For this review, take the finished solid that the model builds, in its own axes (mm). A direction names the side the tool comes from. Give positions to 0.01 mm unless a question says otherwise; leave off trailing zeros. Write each loop counter-clockwise with the first axis right and the second up, starting at its lowest first coordinate (ties: lowest second). Pieces come first, ordered by that corner, then holes. Notation, with made-up numbers: M -33,-12.75 L 24,-12.75 A5 cw 24,-6.75 Z; hole C 37,87 d2. An arc over 180 degrees is marked long. One line per item, written item: value. Start each with the question number.
Item 1: Mouldability with a two-part tool opening along X and no side actions: class faces 1 (the face through (-256.7, 5.1, 83.7)), 2 (the face through (231.62, 16.99, 93.29)), 3 (the face through (23, 0, 4)) as released by +X, released by -X, zero draft, split by the parting line, or undercut.
Item 2: Clearance check with flat-ended pins moving along their axes: pin 1 Ø16.5 at (x, z) = (-234.5, 78.5) entering from +Y; pin 2 Ø5 at (x, y) = (-204.5, 69) entering from -Z; pin 3 Ø14.5 at (x, z) = (-164, 57) entering from +Y; pin 4 Ø11.5 at (x, z) = (-143.49, -197.5) entering from -Y. State where each tip first meets the part, or that it passes through.
Item 3: Tool access review of faces 4 (the face through (139, 20, -191)), 5 (the face through (111.363, 125.695, -124.104)), 6 (the face through (152.443, 125.695, 67.563)): name each direction out of +Z, -Z, +X, -X, +Y, -Y from which nothing blocks a thin tool from reaching the whole face with its end or side.
Item 4: To check wall thickness, follow probe 1 along X at (y, z) = (11.5, 0); probe 2 along Z at (x, y) = (114.5, 27); probe 3 along X at (y, z) = (50, 0). State the ranges of each line that lie inside material, in increasing order.
Item 5: Consider section A-A, the plane z = 0. Write out the cut boundary in (x, y).
Item 6: Consider section B-B, the plane x = 47. Write out the cut boundary in (y, z), and give its area (3 significant figures).
```python
from build123d import *

# Parameters (mm, degrees)
CROQUIS4_R              = 150
SALIENTE_EXTRUIR3_DEPTH = 150
CROQUIS7_R              = 130
CORTAR_EXTRUIR1_DEPTH   = 130
SALIENTE_EXTRUIR5_DEPTH = 20
REDONDEO1_R             = 10
MATRIZC1_COUNT          = 5
REDONDEO1_OF_MATRIZC1_R = 10
CROQUIS13_R             = 20
CORTAR_EXTRUIR2_DEPTH   = 406.648747611


with BuildPart() as part:
    # Croquis4 → Saliente-Extruir3 (new body)
    with BuildSketch(Plane(origin=(0, 0, 0), x_dir=(1, 0, 0), z_dir=(0, 1, 0))):
        with Locations(Location((0, 0, 0), (0, 0, 270))):
            Circle(CROQUIS4_R)
    extrude(amount=SALIENTE_EXTRUIR3_DEPTH)

    # Croquis7 → Cortar-Extruir1 (cut)
    with BuildSketch(Plane(origin=(0, 150, 0), x_dir=(1, 0, 0), z_dir=(0, 1, 0))):
        with Locations(Location((0, 0, 0), (0, 0, 270))):
            Circle(CROQUIS7_R)
    extrude(amount=-CORTAR_EXTRUIR1_DEPTH, mode=Mode.SUBTRACT)

    # Croquis8 → Saliente-Extruir5 (add, symmetric)
    with BuildSketch(Plane(origin=(0, 0, 0), x_dir=(0, 0, -1), z_dir=(1, 0, 0))):
        Polygon((-190.212550173, 128.702405531), (-220, 20), (-270, 20), (-270, 0), (-141.546888578, 0), (-141.546888578, 128.702405531), align=None)
    saliente_extruir5 = extrude(amount=SALIENTE_EXTRUIR5_DEPTH, both=True)

    # Redondeo1
    redondeo1_edges = [part.edges().sort_by_distance(p)[0] for p in [
        (20, 128.702405531, 169.436618823),
        (20, 74.351202766, 205.106275086),
        (20, 20, 245),
        (-20, 128.702405531, 169.436618823),
        (0, 128.702405531, 190.212550173),
        (0, 20, 270),
        (-20, 20, 245),
        (0, 20, 220),
        (-20, 74.351202766, 205.106275086),
    ]]
    fillet(redondeo1_edges, radius=REDONDEO1_R)

    # Croquis12 → Refrentado para tornillo con cabeza plana de M81 (revolve, cut)
    with BuildSketch(Plane(origin=(0, 20, 244.12063984), x_dir=(0, 0, 1), z_dir=(1, 0, 0))):
        Polygon((0, 0), (0, 20), (5, 20), (5, 5), (7.5, 5), (7.5, 0.025), (7.525, 0), align=None)
    refrentado_para_tornillo_con_cabeza_plan = revolve(axis=Axis((0, 26.35, 244.12063984), (0, -1, 0)), mode=Mode.SUBTRACT)

    # MatrizC1: Saliente-Extruir5, Refrentado para tornillo con cabeza plana de M81 ×5 about axis
    matrizc1_axis = Axis((0, 0, 0), (0, 1, 0))
    add([saliente_extruir5.rotate(matrizc1_axis, i * 360 / MATRIZC1_COUNT) for i in range(1, MATRIZC1_COUNT)])
    add([refrentado_para_tornillo_con_cabeza_plan.rotate(matrizc1_axis, i * 360 / MATRIZC1_COUNT) for i in range(1, MATRIZC1_COUNT)], mode=Mode.SUBTRACT)

    # Redondeo1 of MatrizC1
    redondeo1_of_matrizc1_edges = [part.edges().sort_by_distance(p)[0] for p in [
        (167.324140318, 128.702405531, 33.33766436),
        (201.247999341, 74.351202766, 44.360194329),
        (239.18918638, 20, 56.688033296),
        (154.963460543, 128.702405531, 71.379925012),
        (180.902885323, 128.702405531, 58.778910547),
        (256.7852594, 20, 83.434588481),
        (226.828506605, 20, 94.730293948),
        (209.232433585, 20, 67.983738762),
        (188.887319566, 74.351202766, 82.402454981),
        (83.412005855, 128.702405531, -148.832809143),
        (104.378103761, 74.351202766, -177.690167244),
        (127.827046924, 20, -209.964868668),
        (115.77268563, 128.702405531, -125.321399051),
        (111.804131793, 128.702405531, -153.885185633),
        (158.702018119, 20, -218.434588481),
        (160.187726699, 20, -186.453458576),
        (129.312755504, 20, -177.983738762),
        (136.738783536, 74.351202766, -154.178757152),
        (-115.77268563, 128.702405531, -125.321399051),
        (-136.738783536, 74.351202766, -154.178757152),
        (-160.187726699, 20, -186.453458576),
        (-83.412005855, 128.702405531, -148.832809143),
        (-111.804131793, 128.702405531, -153.885185633),
        (-158.702018119, 20, -218.434588481),
        (-127.827046924, 20, -209.964868668),
        (-129.312755504, 20, -177.983738762),
        (-104.378103761, 74.351202766, -177.690167244),
        (-154.963460543, 128.702405531, 71.379925012),
        (-188.887319566, 74.351202766, 82.402454981),
        (-226.828506605, 20, 94.730293948),
        (-167.324140318, 128.702405531, 33.33766436),
        (-180.902885323, 128.702405531, 58.778910547),
        (-256.7852594, 20, 83.434588481),
        (-239.18918638, 20, 56.688033296),
        (-209.232433585, 20, 67.983738762),
        (-201.247999341, 74.351202766, 44.360194329),
    ]]
    fillet(redondeo1_of_matrizc1_edges, radius=REDONDEO1_OF_MATRIZC1_R)

    # Croquis13 → Cortar-Extruir2 (cut, through all)
    with BuildSketch(Plane(origin=(0, 0, 0), x_dir=(1, 0, 0), z_dir=(0, 1, 0))):
        with Locations(Location((0, 0, 0), (0, 0, 270))):
            Circle(CROQUIS13_R)
    extrude(amount=CORTAR_EXTRUIR2_DEPTH, mode=Mode.SUBTRACT)


solid = part.part
```
Model answer:
1. face 1: released by -X
1. face 2: undercut
1. face 3: zero draft
2. pin 1: stops at y = 20
2. pin 2: passes through
2. pin 3: stops at y = 128.7
2. pin 4: stops at y = 0
3. face 4: -Z, +X, +Y
3. face 5: +X, +Y
3. face 6: +Z, +Y
4. probe 1: x = -150 to -20, 20 to 150
4. probe 2: z = -184.16 to -123.57, -96.9 to -61.56, 61.56 to 96.9
4. probe 3: x = -150 to -130, 130 to 150
5. outline: M -150,0 L -20,0 L -20,20 L -130,20 L -130,150 L -150,150 Z; M 20,0 L 150,0 L 150,150 L 130,150 L 130,20 L 20,20 Z
6. outline: M 0,-142.45 L 150,-142.45 L 150,-121.21 L 20,-121.21 L 20,121.21 L 150,121.21 L 150,142.45 L 0,142.45 Z
6. area: 11,200 mm2
